The listing builds one solid part. Answer for the finished solid, in the listing's coordinates (mm). A direction names the side the tool comes from. Coordinates: 2 decimals unless noted, no trailing zeros. Order: outer loops, then holes, each group sorted by start corner. A loop starts at its lowest first (then second) coordinate and runs counter-clockwise, first axis right, second up. Notation, with made-up numbers: (-12.5, -34.5) -> (46.5, -34.5) arc R25 cw to (46.5, -3.5) -> close; hole circle Ø9 at (0, 20). An arc over 180 degrees is marked (long way). Answer in a Markdown table with one row per item.
```python
from build123d import *

# Parameters (mm, degrees)
SKETCH_1_W          = 12
SKETCH_1_H          = 8
EXTRUDE_1_DEPTH     = 3
CUT_EXTRUDE_1_DEPTH = 2
SKETCH_3_R          = 1.75
CUT_EXTRUDE_2_DEPTH = 2
SKETCH_4_W          = 2.2
SKETCH_4_H          = 8
EXTRUDE_2_DEPTH     = 8
FILLET_1_R          = 4
SKETCH_5_R          = 1.75
CUT_EXTRUDE_3_DEPTH = 17.763054614
FILLET_2_R          = 1


with BuildPart() as part:
    # Эскиз1 → Бобышка-Вытянуть1 (new body)
    with BuildSketch(Plane.XY):
        Rectangle(SKETCH_1_W, SKETCH_1_H)
    extrude(amount=EXTRUDE_1_DEPTH)

    # Эскиз2 → Вырез-Вытянуть1 (cut)
    with BuildSketch(Plane.XY.offset(3)):
        Polygon((2.825, -1.63101451), (2.825, 1.63101451), (0, 3.262029021), (-2.825, 1.63101451), (-2.825, -1.63101451), (0, -3.262029021), align=None)
    extrude(amount=-CUT_EXTRUDE_1_DEPTH, mode=Mode.SUBTRACT)

    # Эскиз3 → Вырез-Вытянуть2 (cut)
    with BuildSketch(Plane.XY.offset(1)):
        Circle(SKETCH_3_R)
    extrude(amount=-CUT_EXTRUDE_2_DEPTH, mode=Mode.SUBTRACT)

    # Эскиз4 → Бобышка-Вытянуть2 (add)
    with BuildSketch(Plane.XY.offset(3)):
        with Locations((-4.9, 0)):
            Rectangle(SKETCH_4_W, SKETCH_4_H)
        with Locations((4.9, 0)):
            Rectangle(SKETCH_4_W, SKETCH_4_H)
    extrude(amount=EXTRUDE_2_DEPTH)

    # Скругление1
    fillet_1_edges = [part.edges().sort_by_distance(p)[0] for p in [
        (4.9, 4, 11),
        (-4.9, 4, 11),
        (4.9, -4, 11),
        (-4.9, -4, 11),
    ]]
    fillet(fillet_1_edges, radius=FILLET_1_R - 0.0001)  # a hair under: the kernel refuses the full size

    # Эскиз5 → Вырез-Вытянуть3 (cut, through all)
    with BuildSketch(Plane(origin=(6, 0, 0), x_dir=(0, 0, -1), z_dir=(1, 0, 0))):
        with Locations(Location((-7, 0, 0), (0, 0, 90))):
            Circle(SKETCH_5_R)
    extrude(amount=-CUT_EXTRUDE_3_DEPTH, mode=Mode.SUBTRACT)

    # Скругление2
    fillet_2_edges = [part.edges().sort_by_distance(p)[0] for p in [
        (-3.8, 0, 3),
        (3.8, 0, 3),
    ]]
    fillet(fillet_2_edges, radius=FILLET_2_R)


solid = part.part
```
(1) For a pull along Z with two mould halves and no side action, classify faces 4 (the cylindrical face through (3.499, -2.806, 3.285)), 5 (the cylindrical face through (-4.88, -0.38, 5.29)), 6 (the flat face through (2.825, 0, 2)) as released by +Z, released by -Z, zero draft, split by the parting line, or undercut.
Check values:
| item | result |
|---|---|
| face 4 | released by +Z |
| face 5 | undercut |
| face 6 | zero draft |
(2) Which of the six approach directions +Z, -Z, +X, -X, +Y, -Y give full straight-line access (tool end or side, diameter ignored) to faces 1 (the cylindrical face through (-3.515, -2.806, 3.301)), 2 (the flat face through (1.39, -2.46, 2.01)), 3 (the cylindrical face through (4.915, 2.797, 9.859))?
Check values:
| item | result |
|---|---|
| face 1 | +Z, +Y, -Y |
| face 2 | +Z |
| face 3 | +Z, +X, -X, +Y |
(3) Flat-ended cylindrical pins translate along their axes: pin 1 (1 mm diameter, centred on x = -1.5, y = -1.5, fed in from +Z); pin 2 (1.9 mm diameter, centred on x = -1, y = -3, fed in from +Z); pin 3 (3 mm diameter, centred on x = -1, z = 7.5, fed in from +Y). Find the tip coordinate at first contact, or state that the pin passes through.
Check values:
| item | result |
|---|---|
| pin 1 | z = 1 |
| pin 2 | z = 3 |
| pin 3 | through |
(4) A cutting plane is placed at B-B, the plane z = 5.75. Determine the outline of the cut face in (x, y).
Check values:
| item | result |
|---|---|
| outline | (-6, -4) -> (-3.8, -4) -> (-3.8, -1.22) -> (-6, -1.22) -> close; (-6, 1.22) -> (-3.8, 1.22) -> (-3.8, 4) -> (-6, 4) -> close; (3.8, -4) -> (6, -4) -> (6, -1.22) -> (3.8, -1.22) -> close; (3.8, 1.22) -> (6, 1.22) -> (6, 4) -> (3.8, 4) -> close |
(5) Find the intervals of material crossed by line 1 along X through (y, z) = (-3.25, 5.5); line 2 along X through (y, z) = (-1, 2) (3 decimals); line 3 along Z through (x, y) = (-4.25, 0), in increasing order. Write a range as from..to.
Check values:
| item | result |
|---|---|
| line 1 | -6..-3.8, 3.8..6 |
| line 2 | -6..-2.825, 2.825..6 |
| line 3 | 0..5.25, 8.75..11 |
(6) A cutting plane is placed at D-D, the plane y = 2.5. Determine the outline of the cut face in (x, z), then the cut area to 3 significant figures.
Check values:
| item | result |
|---|---|
| outline | (-6, 0) -> (6, 0) -> (6, 10.12) -> (3.8, 10.12) -> (3.8, 4) arc R1 cw to (2.8, 3) -> (1.32, 3) -> (1.32, 1) -> (-1.32, 1) -> (-1.32, 3) -> (-2.8, 3) arc R1 cw to (-3.8, 4) -> (-3.8, 10.12) -> (-6, 10.12) -> close |
| area | 62.5 mm² |
(7) A cutting plane is placed at C-C, the plane x = -1.25. Determine the outline of the cut face in (y, z), then the cut area to 3 significant figures.
Check values:
| item | result |
|---|---|
| outline | (-4, 0) -> (-1.22, 0) -> (-1.22, 1) -> (-2.54, 1) -> (-2.54, 3) -> (-4, 3) -> close; (1.22, 0) -> (4, 0) -> (4, 3) -> (2.54, 3) -> (2.54, 1) -> (1.22, 1) -> close |
| area | 11.4 mm² |
